The listing builds one solid part. Answer for the finished solid, in the listing's coordinates (mm). Give positions to 0.01 mm unless a question says otherwise; leave off trailing zeros. Write each loop counter-clockwise with the first axis right and the second up, starting at its lowest first coordinate (ties: lowest second). Pieces come first, ordered by that corner, then holes. Notation, with made-up numbers: M 4.5,-10 L 22.5,-10 A19 cw 22.5,4 Z; hole C -2.5,5.25 d10. An arc over 180 degrees is marked long. Answer as a JSON object with one key per item and string values.
```python
from build123d import *

# Parameters (mm, degrees)
F0_R     = 6.5
F1_DEPTH = 6.35


# Not quite as in the source:
# - a length typed as a fraction of an inch, garbled in the dataset ("3 / 203.2 mm" for 3/8 in), is restored


with BuildPart() as f1:
    # F0 (on Top) → F1 (new body)
    with BuildSketch(Plane.XY):
        with BuildLine():
            Line((0, -75), (0, 0))
            Line((0, 0), (-75, 0))
            ThreePointArc((-75, 0), (-68.0942312118, -31.4352616607), (-48.6486486486, -57.0815993527))
            ThreePointArc((-48.6486486486, -57.0815993527), (-25.9218059609, -70.3779793382), (0, -75))
        make_face()
        with BuildLine():
            ThreePointArc((-48.6486486486, -57.0815993527), (-68.0942312118, -31.4352616607), (-75, 0))
            Line((-75, 0), (-77.5, 0))
            ThreePointArc((-77.5, 0), (-86.2129476679, -13.6188462424), (-102.2297297297, -11.4163198705))
            Line((-102.2297297297, -11.4163198705), (-48.6486486486, -57.0815993527))
        make_face()
        with BuildLine():
            Line((-86, 0), (-77.5, 0))
            ThreePointArc((-77.5, 0), (-86.2129476679, 13.6188462424), (-102.2297297297, 11.4163198705))
            ThreePointArc((-102.2297297297, 11.4163198705), (-106.1188462424, 6.2870523321), (-107.5, 0))
            Line((-107.5, 0), (-99, 0))
            ThreePointArc((-99, 0), (-92.5, 6.5), (-86, 0))
        make_face()
        with BuildLine():
            ThreePointArc((48.6486486486, -57.0815993527), (68.0942312118, -31.4352616607), (75, 0))
            Line((75, 0), (0, 0))
            Line((0, 0), (0, -75))
            ThreePointArc((0, -75), (25.9218059609, -70.3779793382), (48.6486486486, -57.0815993527))
        make_face()
        with BuildLine():
            ThreePointArc((-102.2297297297, -11.4163198705), (-86.2129476679, -13.6188462424), (-77.5, 0))
            Line((-77.5, 0), (-86, 0))
            ThreePointArc((-86, 0), (-92.5, -6.5), (-99, 0))
            Line((-99, 0), (-107.5, 0))
            ThreePointArc((-107.5, 0), (-106.1188462424, -6.2870523321), (-102.2297297297, -11.4163198705))
        make_face()
        with BuildLine():
            ThreePointArc((0, 75), (25.9218059609, 70.3779793382), (48.6486486486, 57.0815993527))
            Line((48.6486486486, 57.0815993527), (102.2297297297, 11.4163198705))
            ThreePointArc((102.2297297297, 11.4163198705), (106.1188462424, 6.2870523321), (107.5, 0))
            Line((107.5, 0), (107.5, 75))
            Line((107.5, 75), (0, 75))
        make_face()
        with BuildLine():
            ThreePointArc((-48.6486486486, 57.0815993527), (-25.9218059609, 70.3779793382), (0, 75))
            Line((0, 75), (107.5, 75))
            Line((107.5, 75), (107.5, 380))
            ThreePointArc((107.5, 380), (101.6421356237, 394.1421356237), (87.5, 400))
            Line((87.5, 400), (-87.5, 400))
            ThreePointArc((-87.5, 400), (-101.6421356237, 394.1421356237), (-107.5, 380))
            Line((-107.5, 380), (-107.5, 0))
            ThreePointArc((-107.5, 0), (-106.1188462424, 6.2870523321), (-102.2297297297, 11.4163198705))
            Line((-102.2297297297, 11.4163198705), (-48.6486486486, 57.0815993527))
        make_face()
        with Locations((-87.5, 380)):
            Circle(F0_R, mode=Mode.SUBTRACT)
        with Locations((87.5, 380)):
            Circle(F0_R, mode=Mode.SUBTRACT)
        with BuildLine():
            Line((86, 0), (77.5, 0))
            ThreePointArc((77.5, 0), (86.2129476679, -13.6188462424), (102.2297297297, -11.4163198705))
            ThreePointArc((102.2297297297, -11.4163198705), (106.1188462424, -6.2870523321), (107.5, 0))
            Line((107.5, 0), (99, 0))
            ThreePointArc((99, 0), (92.5, -6.5), (86, 0))
        make_face()
        with BuildLine():
            ThreePointArc((102.2297297297, 11.4163198705), (86.2129476679, 13.6188462424), (77.5, 0))
            Line((77.5, 0), (86, 0))
            ThreePointArc((86, 0), (92.5, 6.5), (99, 0))
            Line((99, 0), (107.5, 0))
            ThreePointArc((107.5, 0), (106.1188462424, 6.2870523321), (102.2297297297, 11.4163198705))
        make_face()
        with BuildLine():
            ThreePointArc((48.6486486486, 57.0815993527), (68.0942312118, 31.4352616607), (75, 0))
            Line((75, 0), (77.5, 0))
            ThreePointArc((77.5, 0), (86.2129476679, 13.6188462424), (102.2297297297, 11.4163198705))
            Line((102.2297297297, 11.4163198705), (48.6486486486, 57.0815993527))
        make_face()
        with BuildLine():
            Line((77.5, 0), (75, 0))
            ThreePointArc((75, 0), (68.0942312118, -31.4352616607), (48.6486486486, -57.0815993527))
            Line((48.6486486486, -57.0815993527), (102.2297297297, -11.4163198705))
            ThreePointArc((102.2297297297, -11.4163198705), (86.2129476679, -13.6188462424), (77.5, 0))
        make_face()
        with BuildLine():
            Line((0, 0), (75, 0))
            ThreePointArc((75, 0), (68.0942312118, 31.4352616607), (48.6486486486, 57.0815993527))
            ThreePointArc((48.6486486486, 57.0815993527), (25.9218059609, 70.3779793382), (0, 75))
            Line((0, 75), (0, 0))
        make_face()
        with BuildLine():
            Line((-77.5, 0), (-75, 0))
            ThreePointArc((-75, 0), (-68.0942312118, 31.4352616607), (-48.6486486486, 57.0815993527))
            Line((-48.6486486486, 57.0815993527), (-102.2297297297, 11.4163198705))
            ThreePointArc((-102.2297297297, 11.4163198705), (-86.2129476679, 13.6188462424), (-77.5, 0))
        make_face()
        with BuildLine():
            Line((-75, 0), (0, 0))
            Line((0, 0), (0, 75))
            ThreePointArc((0, 75), (-25.9218059609, 70.3779793382), (-48.6486486486, 57.0815993527))
            ThreePointArc((-48.6486486486, 57.0815993527), (-68.0942312118, 31.4352616607), (-75, 0))
        make_face()
    extrude(amount=F1_DEPTH)


solid = f1.part
```
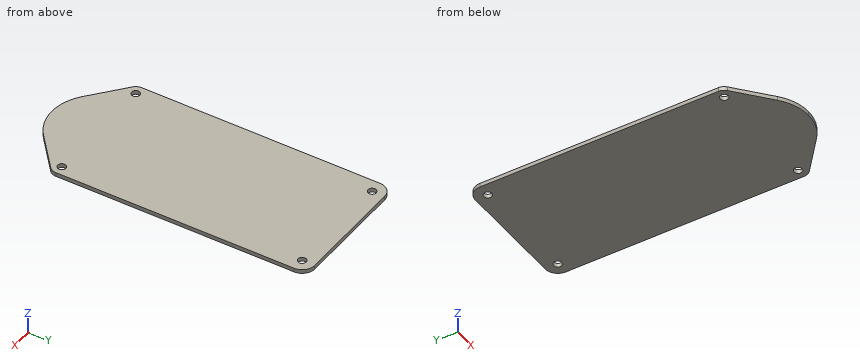
1. Consider line 1 along X through (y, z) = (380, 4); line 2 along X through (y, z) = (6, 1.25); line 3 along Y through (x, z) = (87.5, 3.75). Determine where each line is inside the solid, lowest interval first.
Verdict:
{"line 1": "x = -107.5 to -94, -81 to 81, 94 to 107.5", "line 2": "x = -107.5 to -95, -90 to 90, 95 to 107.5", "line 3": "y = -23.97 to -4.15, 4.15 to 373.5, 386.5 to 400"}
2. Flat-ended cylindrical pins translate along their axes: pin 1 (1 mm diameter, centred on x = -8, z = 1, fed in from -Y); pin 2 (3 mm diameter, centred on x = 76.5, z = 0.5, fed in from -Y). Find the tip coordinate at first contact, or state that the pin passes through.
Verdict:
{"pin 1": "stops at y = -74.62", "pin 2": "stops at y = -34.62"}
3. A cutting plane is placed at A-A, the plane z = 4.5. Give the vertices of the cut face in (x, y), plus the area to 3 significant figures.
Verdict:
{"outline": "M -107.5,0 A15 ccw -102.23,-11.42 L -48.65,-57.08 A75 ccw 48.65,-57.08 L 102.23,-11.42 A15 ccw 107.5,0 L 107.5,380 A20 ccw 87.5,400 L -87.5,400 A20 ccw -107.5,380 Z; hole C -92.5,0 d13; hole C -87.5,380 d13; hole C 87.5,380 d13; hole C 92.5,0 d13", "area": "95,800 mm2"}
4. A cutting plane is placed at C-C, the plane x = 60.5. Give the vertices of the cut face in (y, z), plus the area to 3 significant figures.
Verdict:
{"outline": "M -46.98,0 L 400,0 L 400,6.35 L -46.98,6.35 Z", "area": "2,840 mm2"}
5. A cutting plane is placed at B-B, the plane x = -33.5. Give the vertices of the cut face in (y, z), plus the area to 3 significant figures.
Verdict:
{"outline": "M -67.1,0 L 400,0 L 400,6.35 L -67.1,6.35 Z", "area": "2,970 mm2"}
